Geometry check sheet. Reference: the model listing, model coordinates, mm. A direction names the side the tool comes from. Coordinates: 2 decimals unless noted, no trailing zeros. Write each loop counter-clockwise with the first axis right and the second up, starting at its lowest first coordinate (ties: lowest second). Pieces come first, ordered by that corner, then holes. Notation, with made-up numbers: (-21, -15.75) -> (31, -15.75) arc R18 ccw to (31, -5.75) -> close; hole circle Ø6 at (-20, -2.75). An arc over 180 degrees is marked (long way). Use a Markdown table: item, result.
```python
from build123d import *

# Parameters (mm, degrees)
SKETCH2_W           = 37
SKETCH2_H           = 18.86
BOSS_EXTRUDE1_DEPTH = 11.2
FILLET1_R           = 4.85
BOSS_EXTRUDE2_DEPTH = 11.2
BOSS_EXTRUDE3_DEPTH = 13.3
CUT_EXTRUDE1_DEPTH  = 2.5
FILLET2_R           = 0.8
FILLET3_R           = 2.1
CUT_EXTRUDE2_DEPTH  = 6.5
BOSS_EXTRUDE5_DEPTH = 8.93
SKETCH11_R          = 1.04
CUT_EXTRUDE4_DEPTH  = 8.93
CUT_EXTRUDE5_REACH  = 29.79
SKETCH12_R          = 1.575
SKETCH13_R          = 2.4
CUT_EXTRUDE6_DEPTH  = 1.85
SKETCH14_R          = 1
CUT_EXTRUDE7_DEPTH  = 10


with BuildPart() as part:
    # Sketch2 → Boss-Extrude1 (new body, symmetric)
    with BuildSketch(Plane(origin=(0, 0, 0), x_dir=(0, 0, -1), z_dir=(1, 0, 0))):
        Rectangle(SKETCH2_W, SKETCH2_H)
    extrude(amount=BOSS_EXTRUDE1_DEPTH, both=True)

    # Fillet1
    fillet1_edges = [part.edges().sort_by_distance(p)[0] for p in [
        (11.2, 0, 18.5),
        (-11.2, 0, 18.5),
    ]]
    fillet(fillet1_edges, radius=FILLET1_R)

    # Sketch3 → Boss-Extrude2 (add)
    with BuildSketch(Plane(origin=(0, 0, -18.5), x_dir=(-1, 0, 0), z_dir=(0, 0, -1))):
        with BuildLine():
            Line((-2.65, 7.67), (2.65, 7.67))
            ThreePointArc((2.65, 7.67), (11.2, -0.88), (2.65, -9.43))
            Line((2.65, -9.43), (-2.65, -9.43))
            ThreePointArc((-2.65, -9.43), (-11.2, -0.88), (-2.65, 7.67))
        make_face()
    extrude(amount=BOSS_EXTRUDE2_DEPTH)

    # Sketch4 → Boss-Extrude3 (add)
    with BuildSketch(Plane(origin=(0, 0, -29.7), x_dir=(-1, 0, 0), z_dir=(0, 0, -1))):
        with BuildLine():
            Line((-2.65, -7.96), (2.65, -7.96))
            ThreePointArc((2.65, -7.96), (9.73, -0.88), (2.65, 6.2))
            Line((2.65, 6.2), (-2.65, 6.2))
            ThreePointArc((-2.65, 6.2), (-9.73, -0.88), (-2.65, -7.96))
        make_face()
    extrude(amount=BOSS_EXTRUDE3_DEPTH)

    # Sketch5 → Cut-Extrude1 (cut)
    with BuildSketch(Plane(origin=(0, 0, -43), x_dir=(-1, 0, 0), z_dir=(0, 0, -1))):
        with BuildLine():
            Line((-2.65, -7.96), (2.65, -7.96))
            ThreePointArc((2.65, -7.96), (9.73, -0.88), (2.65, 6.2))
            Line((2.65, 6.2), (-2.65, 6.2))
            ThreePointArc((-2.65, 6.2), (-9.73, -0.88), (-2.65, -7.96))
        make_face()
        with BuildLine():
            Line((-3, 3.12), (3, 3.12))
            ThreePointArc((3, 3.12), (0, -5.88), (-3, 3.12))
        make_face(mode=Mode.SUBTRACT)
    extrude(amount=-CUT_EXTRUDE1_DEPTH, mode=Mode.SUBTRACT)

    # Fillet2
    fillet2_edges = [part.edges().sort_by_distance(p)[0] for p in [
        (0, -5.88, -43),
        (0, 3.12, -43),
    ]]
    fillet(fillet2_edges, radius=FILLET2_R)

    # Fillet3
    fillet3_edges = [part.edges().sort_by_distance(p)[0] for p in [
        (9.73, -0.88, -40.5),
        (0, 6.2, -40.5),
        (-9.73, -0.88, -40.5),
        (0, -7.96, -40.5),
    ]]
    fillet(fillet3_edges, radius=FILLET3_R)

    # Sketch6 → Cut-Extrude2 (cut)
    with BuildSketch(Plane(origin=(0, 0, -40.5), x_dir=(-1, 0, 0), z_dir=(0, 0, -1))):
        with BuildLine():
            Line((9.13, 0.62), (11.2, 0.62))
            ThreePointArc((11.2, 0.62), (12.7, -0.88), (11.2, -2.38))
            Line((11.2, -2.38), (9.13, -2.38))
            ThreePointArc((9.13, -2.38), (7.63, -0.88), (9.13, 0.62))
        make_face()
    cut_extrude2 = extrude(amount=-CUT_EXTRUDE2_DEPTH, mode=Mode.SUBTRACT)

    # Mirror1: Cut-Extrude2 across plane
    add(cut_extrude2.mirror(Plane(origin=(0, 0, 0), x_dir=(0, 0, 1), z_dir=(1, 0, 0))), mode=Mode.SUBTRACT)

    # Sketch10 → Boss-Extrude5 (add)
    with BuildSketch(Plane(origin=(0, 9.43, 0), x_dir=(1, 0, 0), z_dir=(0, 1, 0))):
        with BuildLine():
            Line((-1.915561651, -8.86), (2.135561651, -8.86))
            ThreePointArc((2.135561651, -8.86), (2.86, -7), (2.135561651, -5.14))
            Line((2.135561651, -5.14), (-1.915561651, -5.14))
            ThreePointArc((-1.915561651, -5.14), (-2.64, -7), (-1.915561651, -8.86))
        make_face()
    boss_extrude5 = extrude(amount=BOSS_EXTRUDE5_DEPTH)

    # Sketch11 → Cut-Extrude4 (cut)
    with BuildSketch(Plane(origin=(0, 18.36, 0), x_dir=(1, 0, 0), z_dir=(0, 1, 0))):
        with Locations((0.11, -7)):
            Circle(SKETCH11_R)
    cut_extrude4 = extrude(amount=-CUT_EXTRUDE4_DEPTH, mode=Mode.SUBTRACT)

    # Mirror3: Boss-Extrude5, Cut-Extrude4 across plane
    add(boss_extrude5.mirror(Plane.ZX))
    add(cut_extrude4.mirror(Plane.ZX), mode=Mode.SUBTRACT)

    # Sketch12 → Cut-Extrude5 (cut, up to next)
    with BuildSketch(Plane.XZ.offset(9.43), mode=Mode.PRIVATE) as cut_extrude5_sk1:
        with Locations((8.861437687, -13)):
            Circle(SKETCH12_R)
    cut_extrude5_tool1 = extrude(cut_extrude5_sk1.sketch, amount=-CUT_EXTRUDE5_REACH, mode=Mode.PRIVATE) & part.part
    add(cut_extrude5_tool1.solids().sort_by_distance((8.861438, -9.43, -13))[0], mode=Mode.SUBTRACT)
    # Sketch12 → Cut-Extrude5 (cut, up to next)
    with BuildSketch(Plane.XZ.offset(9.43), mode=Mode.PRIVATE) as cut_extrude5_sk2:
        with Locations((-8.638562313, -13)):
            Circle(SKETCH12_R)
    cut_extrude5_tool2 = extrude(cut_extrude5_sk2.sketch, amount=-CUT_EXTRUDE5_REACH, mode=Mode.PRIVATE) & part.part
    add(cut_extrude5_tool2.solids().sort_by_distance((-8.638562, -9.43, -13))[0], mode=Mode.SUBTRACT)

    # Sketch13 → Cut-Extrude6 (cut)
    with BuildSketch(Plane(origin=(0, 9.43, 0), x_dir=(1, 0, 0), z_dir=(0, 1, 0))):
        with Locations((6.14, 15.7)):
            Circle(SKETCH13_R)
        with Locations((-6.13, 15.7)):
            Circle(SKETCH13_R)
    extrude(amount=-CUT_EXTRUDE6_DEPTH, mode=Mode.SUBTRACT)

    # Sketch14 → Cut-Extrude7 (cut)
    with BuildSketch(Plane(origin=(0, 7.58, 0), x_dir=(1, 0, 0), z_dir=(0, 1, 0))):
        with Locations((-6.13, 15.7)):
            Circle(SKETCH14_R)
        with Locations((6.14, 15.7)):
            Circle(SKETCH14_R)
    extrude(amount=-CUT_EXTRUDE7_DEPTH, mode=Mode.SUBTRACT)


solid = part.part
```
Item 1: Section check C-C on y = -3.5. Count the separate pieces of the cut face and the enclosed holes in it, then the cut area to 3 significant figures.
Answer block:
| item | result |
|---|---|
| separate pieces | 1 |
| enclosed holes | 2 |
| area | 1,260 mm^2 |
Item 2: Section check A-A on y = -13. Record the boundary of the cut face in (x, z).
Answer block:
| item | result |
|---|---|
| outline | (-1.92, 5.14) -> (2.14, 5.14) arc R2.75 ccw to (2.14, 8.86) -> (-1.92, 8.86) arc R2.75 ccw to start; hole circle Ø2.08 at (0.11, 7) |
Item 3: Thickness scan on L1, parallel to X at y = 4, z = -13; L2, parallel to Z at x = 0.11, y = -11.75; L3, parallel to Z at x = -6.13, y = 0. Record the ranges inside material, lowest first. Write a range as [from, to].
Answer block:
| item | result |
|---|---|
| L1 | x = [-11.2, -10.21], [-7.06, 7.29], [10.44, 11.2] |
| L2 | z = [5.14, 5.96], [8.04, 8.86] |
| L3 | z = [-40.5, -16.7], [-14.7, 18.5] |
Item 4: Depth check by flat-ended pin: P1, Ø0.9, axis at x = -0.5, z = -41.5, coming from the +Y side; P2, Ø10, axis at x = -3, y = 10, coming from the -Z side; P3, Ø1, axis at x = -7, z = -1.5, coming from the -Y side; P4, Ø3, axis at x = -8.64, z = -13, coming from the -Y side. Enter the tip coordinate at first touch or a pass-through.
Answer block:
| item | result |
|---|---|
| P1 | stops at y = 3.12 |
| P2 | stops at z = -40.29 |
| P3 | stops at y = -9.43 |
| P4 | passes through |
Item 5: Tool access check on faces 1 (the cylindrical face through (-11.2, -0.7, -24)), 2 (the cylindrical face through (-0.175, -5.877, -41.362)), 3 (the flat face through (-6, -2.42, -16)). Record the directions out of +Z, -Z, +X, -X, +Y, -Y that give a thin tool (end or side, any length) a straight path to the whole face; none if there is none.
Answer block:
| item | result |
|---|---|
| face 1 | -Z, -X |
| face 2 | -Z |
| face 3 | +Y |
Item 6: Section check D-D on z = -33. Record the boundary of the cut face in (x, y), then the cut area to 3 significant figures.
Answer block:
| item | result |
|---|---|
| outline | (-2.65, -7.96) -> (2.65, -7.96) arc R7.08 ccw to (2.65, 6.2) -> (-2.65, 6.2) arc R7.08 ccw to start |
| area | 233 mm^2 |
Item 7: Section check B-B on z = -15.7. Record the boundary of the cut face in (x, y), then the cut area to 3 significant figures.
Answer block:
| item | result |
|---|---|
| outline | (-11.2, -9.43) -> (11.2, -9.43) -> (11.2, 9.43) -> (8.54, 9.43) -> (8.54, 7.58) -> (7.14, 7.58) -> (7.14, -2.42) -> (5.14, -2.42) -> (5.14, 7.58) -> (3.74, 7.58) -> (3.74, 9.43) -> (-3.73, 9.43) -> (-3.73, 7.58) -> (-5.13, 7.58) -> (-5.13, -2.42) -> (-7.13, -2.42) -> (-7.13, 7.58) -> (-8.53, 7.58) -> (-8.53, 9.43) -> (-11.2, 9.43) -> close |
| area | 365 mm^2 |
Item 8: Mould release check, pull along Z, two halves, no side actions. Record for faces 4 (the flat face through (-9, -8, -18.5)), 5 (the flat face through (0, -7.96, -34)), 6 (the cylindrical face through (-0.115, -13.958, 8.015)), 7 (the flat face through (6, -2.42, -16)): +Z half, -Z half, draft (parallel to the pull), parting line (faces both ways), or undercut.
Answer block:
| item | result |
|---|---|
| face 4 | -Z half |
| face 5 | draft |
| face 6 | undercut |
| face 7 | undercut |
